Can you work these out from the model? Positions are in its coordinate system, mm. Face numbers are marked on the shaded views. Round coordinates to 2 decimals unless told otherwise and drop trailing zeros. Loops run counter-clockwise (first coordinate to the right, second up) from the corner with the lowest first, then second, coordinate; pieces in that order, holes last. Notation, with made-up numbers: (-30, 42) -> (29, 42) arc R20 cw to (29, 53) -> close; hole circle Ø9 at (-39.5, 10). An arc over 180 degrees is marked (long way). Use a Markdown table: item, result.
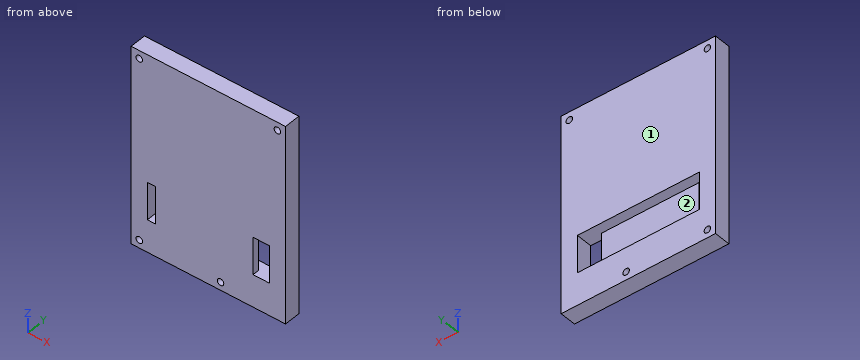
from build123d import *

# Parameters (mm, degrees)
SKETCH_1_W          = 47.5
SKETCH_1_H          = 60.8
EXTRUDE_1_DEPTH     = 5
SKETCH_2_W          = 37.5
SKETCH_2_H          = 11.5
CUT_EXTRUDE_1_DEPTH = 3
SKETCH_3_W          = 2.5
SKETCH_3_H          = 11.5
SKETCH_3_W_2        = 5
CUT_EXTRUDE_2_DEPTH = 2
SKETCH_4_R          = 1
CUT_EXTRUDE_3_DEPTH = 5


with BuildPart() as part:
    # 草图1 → 凸台-拉伸1 (new body)
    with BuildSketch(Plane(origin=(0, 0, 0), x_dir=(1, 0, 0), z_dir=(0, 1, 0))):
        with Locations((-30.655286344, 2.938237127)):
            Rectangle(SKETCH_1_W, SKETCH_1_H)
    extrude(amount=-EXTRUDE_1_DEPTH)

    # 草图2 → 切除-拉伸1 (cut)
    with BuildSketch(Plane(origin=(0, 0, 0), x_dir=(1, 0, 0), z_dir=(0, 1, 0))):
        with Locations((-30.655286344, 17.588237127)):
            Rectangle(SKETCH_2_W, SKETCH_2_H)
    extrude(amount=-CUT_EXTRUDE_1_DEPTH, mode=Mode.SUBTRACT)

    # 草图3 → 切除-拉伸2 (cut)
    with BuildSketch(Plane(origin=(0, -3, 0), x_dir=(1, 0, 0), z_dir=(0, 1, 0))):
        with Locations((-48.155286344, 17.588237127)):
            Rectangle(SKETCH_3_W, SKETCH_3_H)
        with Locations((-14.405286344, 17.588237127)):
            Rectangle(SKETCH_3_W_2, SKETCH_3_H)
    extrude(amount=-CUT_EXTRUDE_2_DEPTH, mode=Mode.SUBTRACT)

    # 草图4 → 切除-拉伸3 (cut)
    with BuildSketch(Plane(origin=(0, 0, 0), x_dir=(1, 0, 0), z_dir=(0, 1, 0))):
        with Locations(Location((-9.405286344, -24.961762873, 0), (0, 0, 270))):
            Circle(SKETCH_4_R)
        with Locations(Location((-51.905286344, -24.961762873, 0), (0, 0, 270))):
            Circle(SKETCH_4_R)
        with Locations(Location((-51.905286344, 30.838237127, 0), (0, 0, 270))):
            Circle(SKETCH_4_R)
        with Locations(Location((-26.905286344, 30.838237127, 0), (0, 0, 270))):
            Circle(SKETCH_4_R)
    extrude(amount=-CUT_EXTRUDE_3_DEPTH, mode=Mode.SUBTRACT)


solid = part.part
1. I want a section at B-B (y = -4.1). Please give me the cut outline in (x, z).
Answer sheet:
| item | result |
|---|---|
| outline | (-54.41, -33.34) -> (-6.91, -33.34) -> (-6.91, 27.46) -> (-54.41, 27.46) -> close; hole circle Ø2 at (-51.91, -30.84); hole circle Ø2 at (-51.91, 24.96); hole (-49.41, -23.34) -> (-46.91, -23.34) -> (-46.91, -11.84) -> (-49.41, -11.84) -> close; hole circle Ø2 at (-26.91, -30.84); hole (-16.91, -23.34) -> (-11.91, -23.34) -> (-11.91, -11.84) -> (-16.91, -11.84) -> close; hole circle Ø2 at (-9.41, 24.96) |
2. Will this pin go through, and if not, where does the flat tip stop? pin 1 Ø1.2 at (x, z) = (-26.91, -30.84) entering from +Y.
Answer sheet:
| item | result |
|---|---|
| pin 1 | passes through |
3. I want a section at D-D (x = -36.5). Please give me the cut outline in (y, z), plus the area to 4 significant figures.
Answer sheet:
| item | result |
|---|---|
| outline | (-5, -33.34) -> (0, -33.34) -> (0, -23.34) -> (-3, -23.34) -> (-3, -11.84) -> (0, -11.84) -> (0, 27.46) -> (-5, 27.46) -> close |
| area | 269.5 mm² |
4. I want a section at C-C (y = -0.65). Please give me the cut outline in (x, z).
Answer sheet:
| item | result |
|---|---|
| outline | (-54.41, -33.34) -> (-6.91, -33.34) -> (-6.91, 27.46) -> (-54.41, 27.46) -> close; hole circle Ø2 at (-51.91, -30.84); hole circle Ø2 at (-51.91, 24.96); hole (-49.41, -23.34) -> (-11.91, -23.34) -> (-11.91, -11.84) -> (-49.41, -11.84) -> close; hole circle Ø2 at (-26.91, -30.84); hole circle Ø2 at (-9.41, 24.96) |
5. I want a section at A-A (x = -14.5). Please give me the cut outline in (y, z).
Answer sheet:
| item | result |
|---|---|
| outline | (-5, -33.34) -> (0, -33.34) -> (0, -23.34) -> (-5, -23.34) -> close; (-5, -11.84) -> (0, -11.84) -> (0, 27.46) -> (-5, 27.46) -> close |
6. I need wall thicknesses on line 1 (X direction, y = -2.15, z = -14); line 2 (Z direction, x = -25.5, y = -2.7); line 3 (Z direction, x = -26, y = -1.7). Which ranges of each line are inside material? Lowest first, please.
Answer sheet:
| item | result |
|---|---|
| line 1 | x = -54.41 to -49.41, -11.91 to -6.91 |
| line 2 | z = -33.34 to -23.34, -11.84 to 27.46 |
| line 3 | z = -33.34 to -31.26, -30.41 to -23.34, -11.84 to 27.46 |
7. If we mould it in two halves opening along Z, with no side actions, what happens to the marked faces 1 and 2? For each: +Z half, -Z half, draft (parallel to the pull), parting line (faces both ways), or undercut.
Answer sheet:
| item | result |
|---|---|
| face 1 | draft |
| face 2 | undercut |
